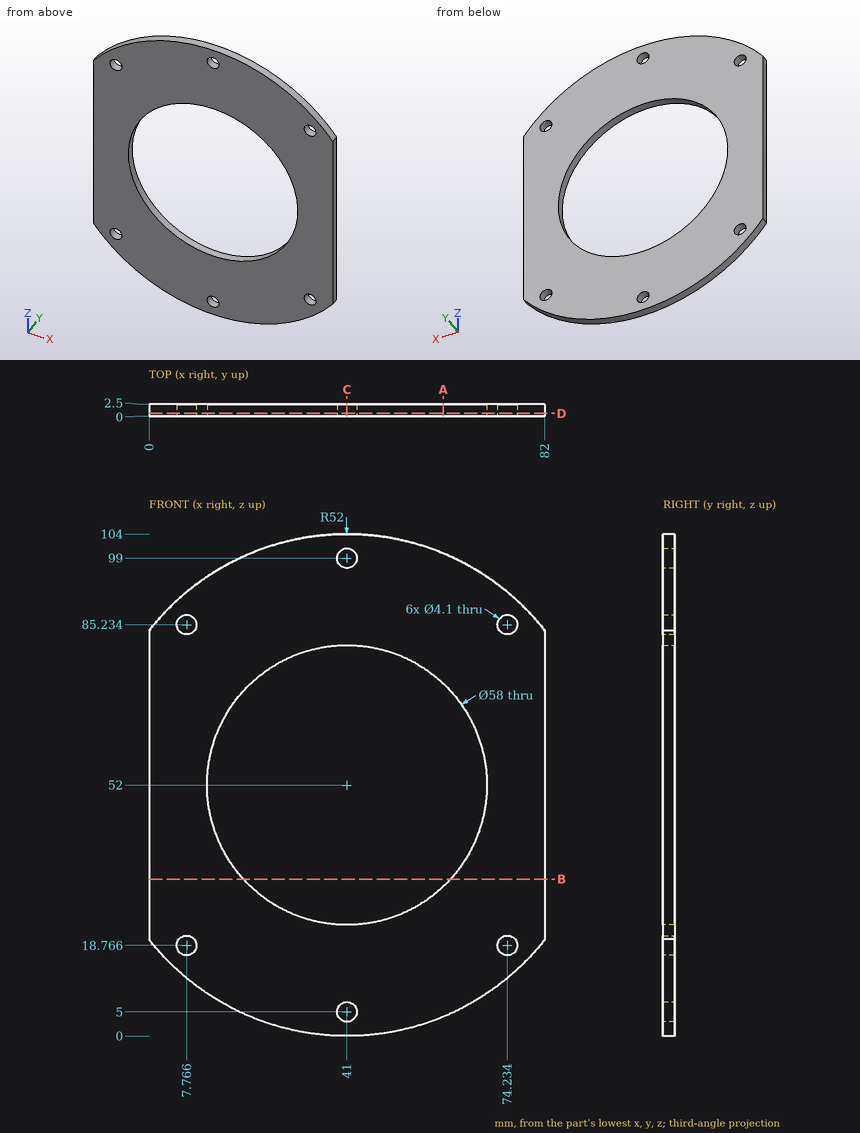
Here's the drawing with two shaded views (mm, measured from the low corner). I have some questions. Coordinates: 2 decimals unless noted, no trailing zeros. Loops run counter-clockwise (first coordinate to the right, second up) from the corner with the lowest first, then second, coordinate; pieces in that order, holes last. Notation, with made-up numbers: M 14,38.5 L 40,38.5 A16 ccw 40,61.5 Z; hole C 87.25,55 d4. An arc over 180 degrees is marked long. Put each result on its own line as item: value. Start each with the question number.
(1) Imagine slicing it at C-C on x = 41. List the corners of the cut face in (y, z) for me.
(2) I need wall thicknesses on probe 1 along X at (y, z) = (0.9, 52); probe 2 along X at (y, z) = (0.35, 28); probe 3 along Z at (x, y) = (23, 0.55). Which ranges of each line are inside material? Lowest first, please.
(3) Imagine slicing it at B-B on z = 32.5. List the corners of the cut face in (x, y) for me, and give its area (3 significant figures).
(4) Will this pin go through, and if not, where does the flat tip stop? pin 1 Ø1 at (x, y) = (31.5, 1.5) entering from -Z.
(5) Imagine slicing it at A-A on x = 61. List the corners of the cut face in (y, z) for me.
(6) Imagine slicing it at D-D on y = 0.55. List the corners of the cut face in (x, z) for me.
Worked answers:
1. outline: M 0,0 L 2.5,0 L 2.5,2.95 L 0,2.95 Z; M 0,7.05 L 2.5,7.05 L 2.5,23 L 0,23 Z; M 0,81 L 2.5,81 L 2.5,96.95 L 0,96.95 Z; M 0,101.05 L 2.5,101.05 L 2.5,104 L 0,104 Z
2. probe 1: x = 0 to 12, 70 to 82
2. probe 2: x = 0 to 24.72, 57.28 to 82
2. probe 3: z = 3.21 to 29.26, 74.74 to 100.79
3. outline: M 0,0 L 19.53,0 L 19.53,2.5 L 0,2.5 Z; M 62.47,0 L 82,0 L 82,2.5 L 62.47,2.5 Z
3. area: 97.7 mm2
4. pin 1: stops at z = 0.78
5. outline: M 0,4 L 2.5,4 L 2.5,31 L 0,31 Z; M 0,73 L 2.5,73 L 2.5,100 L 0,100 Z
6. outline: M 0,20.02 A52 ccw 82,20.02 L 82,83.98 A52 ccw 0,83.98 Z; hole C 7.77,18.77 d4.1; hole C 7.77,85.23 d4.1; hole C 41,52 d58; hole C 41,5 d4.1; hole C 41,99 d4.1; hole C 74.23,18.77 d4.1; hole C 74.23,85.23 d4.1
